Can you work these out from the model? Positions are in its coordinate system, mm. Face numbers are marked on the shaded views. Round coordinates to 2 decimals unless told otherwise and drop trailing zeros. Order: outer loops, then holes, each group sorted by start corner. A loop starts at its lowest first (then second) coordinate and runs counter-clockwise, first axis right, second up.
Q1. Will these pins go through, and if not, where does the flat tip stop? P1, Ø3, axis at x = 20.5, z = 428.5, coming from the -Y side; P2, Ø4, axis at x = 186.5, z = 462.5, coming from the +Y side; P3, Ø2, axis at x = 82.5, y = -140.5, coming from the -Z side.
Q2. If we section it at B-B (z = 294): Please give me the cut outline in (x, y), plus the area to 3 significant figures.
Q3. If we section it at D-D (x = 57): Please give me the cut outline in (y, z), plus the area to 3 significant figures.
Q4. If I drill on line 1 (X direction, y = -254.5, z = 158); line 2 (Z direction, x = 135, y = -188.5); line 3 (Z direction, x = 185.5, y = -312.5), over which ranges is the centre line in solid material (lowest first)?
Q5. If we section it at C-C (x = 23): Please give me the cut outline in (y, z).
Q6. If we section it at A-A (y = -277): Please give me the cut outline in (x, z), plus the area to 3 significant figures.
Q7. We'd pull the mould along X, two halves only. Please class the marked faces 1, 2, 3 and 4: pulls with the +X half, pulls with the -X half, needs draft (parallel to the pull), parting line crosses it, or undercut.
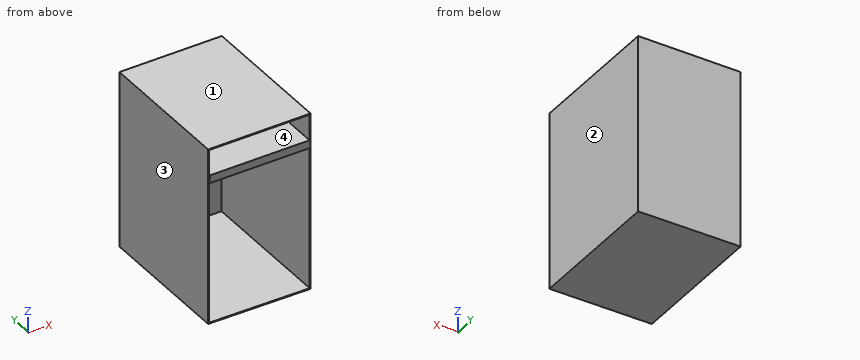
from build123d import *

# Parameters (mm, degrees)
F1_DEPTH = 381
F2_T     = -2.54
F4_DEPTH = 381


with BuildPart() as f1:
    # F0 (on Front) → F1 (new body)
    with BuildSketch(Plane.XZ):
        Polygon((-49.257257, 553.153683), (-49.257257, 70.553683), (230.142743, 68.222205), (230.142743, 553.153683), align=None)
    extrude(amount=F1_DEPTH)

    # F2
    f2_openings = [f1.faces().sort_by_distance(p)[0] for p in [
        (90.554956, -381, 311.270346),
    ]]
    offset(amount=F2_T, openings=f2_openings)

    # F3 (on Front) → F4 (join)
    with BuildSketch(Plane.XZ):
        Polygon((227.298021, 479.927242), (-43.756042, 479.927242), (-46.033807, 458.288461), (227.298021, 458.288461), align=None)
    extrude(amount=F4_DEPTH)


solid = f1.part
Solution:
1. P1: stops at y = -2.54
1. P2: stops at y = 0
1. P3: stops at z = 69.45
2. outline: (-49.26, -381) - (-46.72, -381) - (-46.72, -2.54) - (227.6, -2.54) - (227.6, -381) - (230.14, -381) - (230.14, 0) - (-49.26, 0) - close
2. area: 2,630 mm2
3. outline: (-381, 69.67) - (0, 69.67) - (0, 553.15) - (-381, 553.15) - (-381, 550.61) - (-2.54, 550.61) - (-2.54, 479.93) - (-381, 479.93) - (-381, 458.29) - (-2.54, 458.29) - (-2.54, 72.21) - (-381, 72.21) - close
3. area: 11,300 mm2
4. line 1: x = -49.26 to -46.72, 227.6 to 230.14
4. line 2: z = 69.02 to 71.56, 458.29 to 479.93, 550.61 to 553.15
4. line 3: z = 68.59 to 71.13, 458.29 to 479.93, 550.61 to 553.15
5. outline: (-381, 69.95) - (0, 69.95) - (0, 553.15) - (-381, 553.15) - (-381, 550.61) - (-2.54, 550.61) - (-2.54, 479.93) - (-381, 479.93) - (-381, 458.29) - (-2.54, 458.29) - (-2.54, 72.49) - (-381, 72.49) - close
6. outline: (-49.26, 70.55) - (230.14, 68.22) - (230.14, 553.15) - (-49.26, 553.15) - close; (-46.03, 458.29) - (227.3, 458.29) - (227.3, 479.93) - (-43.76, 479.93) - close; hole (-46.72, 73.07) - (227.6, 70.78) - (227.6, 550.61) - (-46.72, 550.61) - close
6. area: 9,740 mm2
7. face 1: needs draft
7. face 2: pulls with the +X half
7. face 3: pulls with the -X half
7. face 4: undercut
